Build history of the part. All positions in model axes, mm. Face numbers are marked on the shaded views. A direction names the side the tool comes from. Give positions to 0.01 mm unless a question says otherwise; leave off trailing zeros. Loops run counter-clockwise (first coordinate to the right, second up) from the corner with the lowest first, then second, coordinate; pieces in that order, holes last. Notation, with made-up numbers: M -21.5,4 L 5.5,4 A26 ccw 5.5,23 Z; hole C 47,58 d7. An arc over 180 degrees is marked long. Answer in a Markdown table with one row per item. Add a question column.
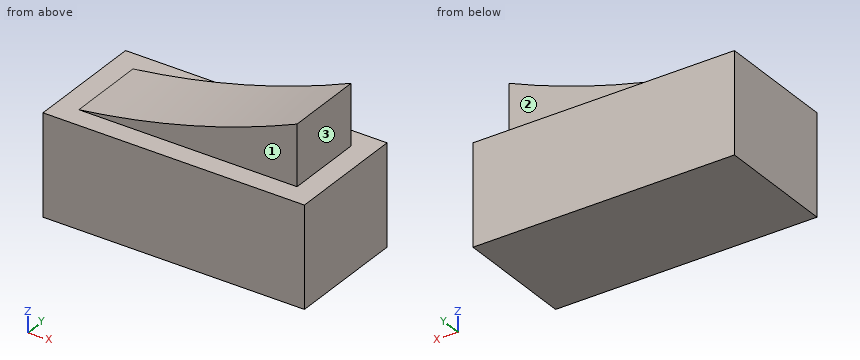
```python
from build123d import *

# Parameters (mm, degrees)
SKETCH1_W           = 6.5
SKETCH1_H           = 2.5
BOSS_EXTRUDE1_DEPTH = 3
SKETCH2_W           = 5.424331786
SKETCH2_H           = 1.966345426
BOSS_EXTRUDE2_DEPTH = 1.5
CUT_EXTRUDE1_DEPTH  = 3.483172713


with BuildPart() as part:
    # Sketch1 → Boss-Extrude1 (new body)
    with BuildSketch(Plane(origin=(0, 0, 0), x_dir=(1, 0, 0), z_dir=(0, 1, 0))):
        Rectangle(SKETCH1_W, SKETCH1_H)
    extrude(amount=BOSS_EXTRUDE1_DEPTH)

    # Sketch2 → Boss-Extrude2 (add)
    with BuildSketch(Plane.XY.offset(1.25)):
        with Locations((0, 1.5)):
            Rectangle(SKETCH2_W, SKETCH2_H)
    extrude(amount=BOSS_EXTRUDE2_DEPTH)

    # Sketch4 → Cut-Extrude1 (cut, through all)
    with BuildSketch(Plane.XZ.offset(-0.516827287)):
        with BuildLine():
            Line((-2.712165893, 2.75), (2.712165893, 2.75))
            ThreePointArc((2.712165893, 2.75), (0.052459338, 1.810295429), (-2.712165893, 1.25))
            Line((-2.712165893, 1.25), (-2.712165893, 2.75))
        make_face()
    extrude(amount=-CUT_EXTRUDE1_DEPTH, mode=Mode.SUBTRACT)


solid = part.part
```
(1) Slice it at C-C, the plane x = -2.25. Give the cut face in (y, z).
(2) Wall check: line 1 (Y direction, x = 1.5, z = 1.3); line 2 (Z direction, x = 2.75, y = 1.9); line 3 (Z direction, x = -0.25, y = 1.55). Give the ranges that are in metal, low to high.
(3) Tool access for the marked faces 1, 2 and 3: list every direction of +Z, -Z, +X, -X, +Y, -Y with a clear straight run to the whole face (end or side of a thin tool).
(4) Slice it at A-A, the plane y = 2.25. Give the cut face in (x, z), then the cut area to 3 significant figures.
(5) Slice it at B-B, the plane x = -0.25. Give the cut face in (y, z).
(6) Slice it at D-D, the plane y = 0.2. Give the cut face in (x, z).
(7) Pin check, flat tips, straight feed: pin 1 (1.5 mm diameter, centred on x = 1, y = 1.5, fed in from +Z); pin 2 (0.8 mm diameter, centred on x = 1, z = 2, fed in from +Y). Stop position of each tip, or through.
Solution:
| question | item | result |
|---|---|---|
| 1 | outline | M 0,-1.25 L 3,-1.25 L 3,1.25 L 2.48,1.25 L 2.48,1.32 L 0.52,1.32 L 0.52,1.25 L 0,1.25 Z |
| 2 | line 1 | 0.52 to 2.48 |
| 2 | line 2 | -1.25 to 1.25 |
| 2 | line 3 | -1.25 to 1.73 |
| 3 | face 1 | +Z, +X, -X, -Y |
| 3 | face 2 | +Z, +X, -X, +Y |
| 3 | face 3 | +Z, +X, +Y, -Y |
| 4 | outline | M -3.25,-1.25 L 3.25,-1.25 L 3.25,1.25 L 2.71,1.25 L 2.71,2.75 A20.21 cw -2.71,1.25 L -3.25,1.25 Z |
| 4 | area | 19.6 mm^2 |
| 5 | outline | M 0,-1.25 L 3,-1.25 L 3,1.25 L 2.48,1.25 L 2.48,1.73 L 0.52,1.73 L 0.52,1.25 L 0,1.25 Z |
| 6 | outline | M -3.25,-1.25 L 3.25,-1.25 L 3.25,1.25 L -3.25,1.25 Z |
| 7 | pin 1 | z = 2.36 |
| 7 | pin 2 | y = 2.48 |
